Source: CAD feature listing. Evaluate the final solid. Frame: model axes, mm. A direction names the side the tool comes from. Round coordinates to 2 decimals unless told otherwise and drop trailing zeros. Order: outer loops, then holes, each group sorted by start corner. A loop starts at its lowest first (then second) coordinate and runs counter-clockwise, first axis right, second up. Notation, with made-up numbers: M 11.5,87 L 22.5,87 A24 cw 22.5,117 Z; hole C 86.25,-13.75 d3. An arc over 180 degrees is marked long. Use one line per item in the form item = value. Start each with the question number.
Q1. Reachability of faces 1 (the flat face through (79, -4, -30)), 2 (the flat face through (79, 11, -64)), 3 (the flat face through (74.5, 32, -66)), 4 (the flat face through (64, 46, -66)), 5 (the flat face through (18, -2, -15)) from +Z, -Z, +X, -X, +Y, -Y: full face, straight path, thin tool, end or side. Return the list, or none.
Q2. Section A-A (x = 94). Return the cut outline in (y, z), plus the area to 3 significant figures.
Q3. Section B-B (z = -13.5). Return the cut outline in (x, y).
Q4. Contact query for flat-ended pins moving along their axis: pin 1 (12 mm diameter, centred on x = 42, y = 21.5, fed in from +Z); pin 2 (6 mm diameter, centred on x = 118.5, z = -17, fed in from +Y). Output: stop coordinate, or through.
Q5. Pull-direction query (X, two-part tool) for faces 6 (the cylindrical face through (80.1, 15.5, -66)), 7 (the flat face through (79, 11, -68)), 8 (the flat face through (27.88, 36.14, -66.03)); classes: pulls with the +X half, pulls with the -X half, needs draft (parallel to the pull), parting line crosses it, or undercut.
Q6. Section D-D (z = -55). Return the cut outline in (x, y).
Q7. Material intervals for probe 1 along Z at (x, y) = (41, 6.5); probe 2 along Y at (x, z) = (143.5, -56); probe 3 along Y at (x, z) = (10, -63), sorted ascending.
Q8. Section C-C (y = 30.5). Return the cut outline in (x, z) (3 decimals).
from build123d import *

# Parameters (mm, degrees)
BASE_FLANGE1_DEPTH      = 4
EDGE_FLANGE1_DEPTH      = 160
EDGE_FLANGE1_START      = -4
EDGE_FLANGE1_FLAT_DEPTH = 4
CHAMFER1_SIZE           = 2


# Sheet-metal steps are written as plain solids
with BuildPart() as part:
    # Sketch1 → Base-Flange1 (new body)
    with BuildSketch(Plane(origin=(0, 0, 0), x_dir=(1, 0, 0), z_dir=(0, 1, 0))):
        with BuildLine():
            Line((0, 0), (18, 0))
            Line((18, 0), (18, 30))
            ThreePointArc((18, 30), (25, 37), (32, 30))
            Line((32, 30), (32, 0))
            Line((32, 0), (128, 0))
            Line((128, 0), (128, 30))
            ThreePointArc((128, 30), (135, 37), (142, 30))
            Line((142, 30), (142, 0))
            Line((142, 0), (160, 0))
            Line((160, 0), (160, 60))
            Line((160, 60), (0, 60))
            Line((0, 60), (0, 0))
        make_face()
    extrude(amount=-BASE_FLANGE1_DEPTH)

    # Edge-Flange1 bend section (across the edge) → Edge-Flange1 (add)
    with BuildSketch(Plane(origin=(160, 0, -64), x_dir=(0, 0, 1), z_dir=(-1, 0, 0))):
        with BuildLine():
            Line((-4, 4), (0, 4))
            ThreePointArc((0, 4), (1.171572875, 1.171572875), (4, 0))
            Line((4, 0), (4, -4))
            ThreePointArc((4, -4), (-1.656854249, -1.656854249), (-4, 4))
        make_face()
    extrude(amount=EDGE_FLANGE1_DEPTH)

    # Edge-Flange1 profile (on flange) → Edge-Flange1 flat (add)
    with BuildSketch(Plane.XY.offset(-64).offset(EDGE_FLANGE1_START)):
        with BuildLine():
            Line((0, 4), (160, 4))
            Line((160, 4), (160, 26))
            Line((160, 26), (105, 46))
            Line((105, 46), (87.5, 46))
            Line((87.5, 46), (85.5, 44))
            Line((85.5, 44), (85.5, 21))
            ThreePointArc((85.5, 21), (80, 15.5), (74.5, 21))
            Line((74.5, 21), (74.5, 44))
            Line((74.5, 44), (72.5, 46))
            Line((72.5, 46), (55, 46))
            Line((55, 46), (0, 26))
            Line((0, 26), (0, 4))
        make_face()
    extrude(amount=EDGE_FLANGE1_FLAT_DEPTH)

    # Chamfer1
    chamfer1_edges = [part.edges().sort_by_distance(p)[0] for p in [
        (160, -2, 0),
        (0, -2, 0),
    ]]
    chamfer(chamfer1_edges, length=CHAMFER1_SIZE)


solid = part.part
Results list:
q1.face_1 = +Z, -Z, +X, -X, -Y
q1.face_2 = +Z, +X, -X, +Y
q1.face_3 = +Z, -Z, +Y
q1.face_4 = +Z, -Z, +X, -X, +Y
q1.face_5 = +Z, +Y, -Y
q2.outline = M -4,-60 A8 ccw 4,-68 L 46,-68 L 46,-64 L 4,-64 A4 cw 0,-60 L 0,0 L -4,0 Z
q2.area = 446 mm2
q3.outline = M 0,-4 L 18,-4 L 18,0 L 0,0 Z; M 32,-4 L 128,-4 L 128,0 L 32,0 Z; M 142,-4 L 160,-4 L 160,0 L 142,0 Z
q4.pin_1 = -64
q4.pin_2 = 0
q5.face_6 = undercut
q5.face_7 = needs draft
q5.face_8 = pulls with the -X half
q6.outline = M 0,-4 L 160,-4 L 160,0 L 0,0 Z
q7.probe_1 = -68 to -64
q7.probe_2 = -4 to 0
q7.probe_3 = -3.42 to 1.35
q8.outline = M 12.375,-68 L 74.5,-68 L 74.5,-64 L 12.375,-64 Z; M 85.5,-68 L 147.625,-68 L 147.625,-64 L 85.5,-64 Z
